Build history of the part. All positions in model axes, mm. A direction names the side the tool comes from. Round coordinates to 2 decimals unless told otherwise and drop trailing zeros. One line per item, written item: value. Start each with the question number.
Item 1: Band-saw the part on A-A, the plane z = 0. Give the number of separate pieces and of enclosed holes in the cut face, then the cut area to 3 significant figures.
Item 2: Probe L1, parallel to X at y = -4.75, z = -33.5 (3 decimals); L2, parallel to Y at x = 4, z = -12.5 (3 decimals); L3, parallel to Y at x = 10.2, z = 101.6. List the from-to ranges inside material, lowest first.
Item 3: Pin check, flat tips, straight feed: pin 1 (6 mm diameter, centred on y = -1, z = 77.5, fed in from +X); pin 2 (15 mm diameter, centred on y = 2.38, z = 32.03, fed in from -X) (3 decimals); pin 3 (1.5 mm diameter, centred on x = 0, z = -75, fed in from +Y) (3 decimals). Stop position of each tip, or through.
Item 4: Tool access for faces 1 (the flat face through (4, -9.525, 2)), 2 (the cylindrical face through (11.09, 3.001, -59.053)): list every direction of +Z, -Z, +X, -X, +Y, -Y with a clear straight run to the whole face (end or side of a thin tool).
Item 5: Two-plate mould, pull along X, no slides. Class faces 3 (the cylindrical face through (-1.349, -11.09, 11.005)), 4 (the flat face through (9.525, 8, 2)), 5 (the cylindrical face through (11.09, 3, -74.93)): +X half, -X half, draft (parallel to the pull), parting line (faces both ways), or undercut.
```python
from build123d import *

# Parameters (mm, degrees)
BOSS_EXTRUDE1_DEPTH = 127
SKETCH4_R           = 1.651
SKETCH4_R_2         = 4.7625
CUT_EXTRUDE1_DEPTH  = 130.554006596
SKETCH5_R           = 1.651
SKETCH5_R_2         = 4.7625
CUT_EXTRUDE2_DEPTH  = 130.554006596


with BuildPart() as part:
    # Sketch2 → Boss-Extrude1 (new, symmetric)
    with BuildSketch(Plane.XY):
        with BuildLine():
            Line((-12.7, -12.7), (12.7, -12.7))
            Line((12.7, -12.7), (12.7, 12.7))
            Line((12.7, 12.7), (11.1125, 12.7))
            ThreePointArc((11.1125, 12.7), (9.989967985, 12.235032015), (9.525, 11.1125))
            Line((9.525, 11.1125), (9.525, -6.35))
            ThreePointArc((9.525, -6.35), (8.59506403, -8.59506403), (6.35, -9.525))
            Line((6.35, -9.525), (-11.1125, -9.525))
            ThreePointArc((-11.1125, -9.525), (-12.235032015, -9.989967985), (-12.7, -11.1125))
            Line((-12.7, -11.1125), (-12.7, -12.7))
        make_face()
    extrude(amount=BOSS_EXTRUDE1_DEPTH, both=True)

    # Sketch4 → Cut-Extrude1 (cut, through all)
    with BuildSketch(Plane(origin=(0, -9.525, 0), x_dir=(1, 0, 0), z_dir=(0, 1, 0))):
        with Locations(Location((-5.55625, 101.6, 0), (0, 0, 180))):
            Circle(SKETCH4_R)
        with Locations(Location((0.79375, 88.907891862, 0), (0, 0, 180))):
            Circle(SKETCH4_R)
        with Locations((0.79375, -88.907891862)):
            Circle(SKETCH4_R)
        with Locations((-5.55625, -101.6)):
            Circle(SKETCH4_R)
        with Locations(Location((-2.38125, 79.662291862, 0), (0, 0, 180))):
            Circle(SKETCH4_R_2)
        with Locations(Location((-2.38125, 63.660291862, 0), (0, 0, 180))):
            Circle(SKETCH4_R_2)
        with Locations(Location((-2.38125, 47.658291862, 0), (0, 0, 180))):
            Circle(SKETCH4_R_2)
        with Locations(Location((-2.38125, 31.656291862, 0), (0, 0, 180))):
            Circle(SKETCH4_R_2)
        with Locations(Location((-2.38125, 15.654291862, 0), (0, 0, 180))):
            Circle(SKETCH4_R_2)
        with Locations(Location((-2.38125, 0, 0), (0, 0, 180))):
            Circle(SKETCH4_R_2)
        with Locations(Location((-2.38125, -15.654291862, 0), (0, 0, 180))):
            Circle(SKETCH4_R_2)
        with Locations(Location((-2.38125, -31.656291862, 0), (0, 0, 180))):
            Circle(SKETCH4_R_2)
        with Locations(Location((-2.38125, -47.658291862, 0), (0, 0, 180))):
            Circle(SKETCH4_R_2)
        with Locations((-2.38125, -63.660291862)):
            Circle(SKETCH4_R_2)
        with Locations((-2.38125, -79.662291862)):
            Circle(SKETCH4_R_2)
    extrude(amount=-CUT_EXTRUDE1_DEPTH, mode=Mode.SUBTRACT)

    # Sketch5 → Cut-Extrude2 (cut, through all)
    with BuildSketch(Plane.ZY.offset(-9.525)):
        with Locations(Location((-88.9, -0.79375, 0), (0, 0, 270))):
            Circle(SKETCH5_R)
        with Locations(Location((-101.6, 5.55625, 0), (0, 0, 270))):
            Circle(SKETCH5_R)
        with Locations(Location((88.9, -0.79375, 0), (0, 0, 90))):
            Circle(SKETCH5_R)
        with Locations(Location((101.6, 5.55625, 0), (0, 0, 90))):
            Circle(SKETCH5_R)
        with Locations(Location((-79.650437411, 2.38125, 0), (0, 0, 270))):
            Circle(SKETCH5_R_2)
        with Locations(Location((-63.775437411, 2.38125, 0), (0, 0, 270))):
            Circle(SKETCH5_R_2)
        with Locations(Location((-47.900437411, 2.38125, 0), (0, 0, 270))):
            Circle(SKETCH5_R_2)
        with Locations(Location((-32.025437411, 2.38125, 0), (0, 0, 270))):
            Circle(SKETCH5_R_2)
        with Locations(Location((-16.150437411, 2.38125, 0), (0, 0, 270))):
            Circle(SKETCH5_R_2)
        with Locations(Location((0, 2.38125, 0), (0, 0, 270))):
            Circle(SKETCH5_R_2)
        with Locations(Location((16.150437411, 2.38125, 0), (0, 0, 90))):
            Circle(SKETCH5_R_2)
        with Locations(Location((32.025437411, 2.38125, 0), (0, 0, 90))):
            Circle(SKETCH5_R_2)
        with Locations(Location((47.900437411, 2.38125, 0), (0, 0, 90))):
            Circle(SKETCH5_R_2)
        with Locations(Location((63.775437411, 2.38125, 0), (0, 0, 90))):
            Circle(SKETCH5_R_2)
        with Locations(Location((79.650437411, 2.38125, 0), (0, 0, 90))):
            Circle(SKETCH5_R_2)
    extrude(amount=-CUT_EXTRUDE2_DEPTH, mode=Mode.SUBTRACT)


solid = part.part
```
Output:
1. separate pieces: 3
1. enclosed holes: 0
1. area: 91.8 mm²
2. L1: x = 9.525 to 12.7
2. L2: y = -12.7 to -9.525
2. L3: y = -12.7 to 3.91, 7.21 to 12.41
3. pin 1: stops at x = 12.7
3. pin 2: stops at x = 9.525
3. pin 3: stops at y = -9.525
4. face 1: +Z, -Z, -X, +Y
4. face 2: +X, -X
5. face 3: undercut
5. face 4: -X half
5. face 5: draft
